Read the model definition and answer for the solid it produces. Units are mm, in the model's axes. Face numbers are marked on the shaded views. A direction names the side the tool comes from. Round coordinates to 2 decimals unless told otherwise and drop trailing zeros. Order: outer loops, then holes, each group sorted by start corner. A loop starts at its lowest first (then second) coordinate and runs counter-clockwise, first axis right, second up. Notation, with made-up numbers: (-20.75, 6.5) - (6.25, 6.5) arc R21 ccw to (6.25, 28.5) - close; hole circle Ø4 at (49.25, 9). An arc over 180 degrees is marked (long way). One line per question, with ' | ' between items. Start each with the question number.
1) The mould has two halves that part along X. Classify the marked faces 6, 7, 8 and 9: pulls with the +X half, pulls with the -X half, needs draft (parallel to the pull), parting line crosses it, or undercut.
2) Flat-ended cylindrical pins translate along their axes: pin 1 (20.5 mm diameter, centred on x = 66.5, y = -26, fed in from -Z); pin 2 (10 mm diameter, centred on x = -58.7, z = 38.1, fed in from -Y) (3 decimals); pin 3 (5 mm diameter, centred on x = -50.5, y = -50, fed in from -Z). Find the tip coordinate at first contact, or state that the pin passes through.
3) The part is cut by section A-A, the plane x = 0. Give the vertices of the cut face in (y, z) (3 decimals), plus the area to 3 significant figures.
4) For the marked faces 1, 2, 3, 4 and 5, determine the directions among +Z, -Z, +X, -X, +Y, -Y from which every point of the face is accessible in a straight line to the end or side of a thin tool.
5) The part is cut by section B-B, the plane z = 0. Give the vertices of the cut face in (x, y) (3 decimals), plus the area to 3 significant figures.
6) The part is cut by section D-D, the plane z = 25. Give the vertices of the cut face in (x, y) (3 decimals).
7) The part is cut by section C-C, the plane y = -20.5. Give the vertices of the cut face in (x, z).
8) Straight lines are drawn through the part: line 1 (X direction, y = -63, z = 38); line 2 (Z direction, x = 67.5, y = -17); line 3 (Y direction, x = -33.5, z = 19.5) (3 decimals). For each, find the intervals that lie inside material, in ascending order. Write a range as from..to.
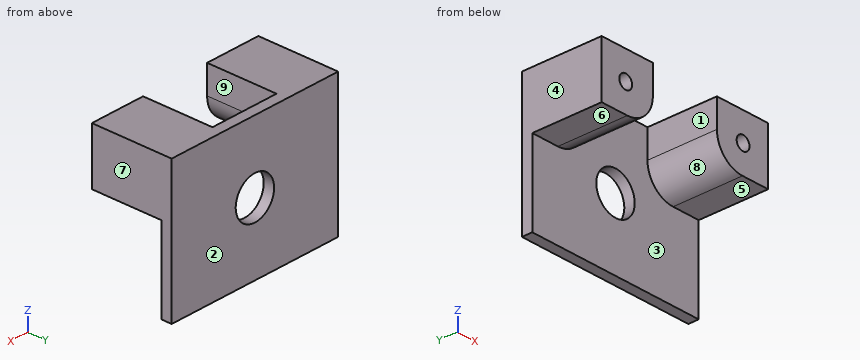
from build123d import *

# Parameters (mm, degrees)
F0_W     = 165.1
F0_H     = 127
F1_DEPTH = 9.525
F3_DEPTH = 63.5
F4_R     = 19.05
F6_DEPTH = 50.8
F5_R     = 6.35
F7_DEPTH = 25.4
F8_R     = 6.35
F9_DEPTH = 25.4


with BuildPart() as f1:
    # F0 (on Front) → F1 (new body)
    with BuildSketch(Plane.XZ):
        Rectangle(F0_W, F0_H)
    extrude(amount=F1_DEPTH)

    # F2 (on face) → F3 (join)
    with BuildSketch(Plane.XZ.offset(9.525)):
        with BuildLine():
            Line((82.55, 63.5), (31.75, 63.5))
            Line((31.75, 63.5), (31.75, 38.1))
            ThreePointArc((31.75, 38.1), (39.189488, 20.139488), (57.15, 12.7))
            Line((57.15, 12.7), (82.55, 12.7))
            Line((82.55, 12.7), (82.55, 63.5))
        make_face()
        with BuildLine():
            Line((-31.75, 63.5), (-82.55, 63.5))
            Line((-82.55, 63.5), (-82.55, 12.7))
            Line((-82.55, 12.7), (-57.15, 12.7))
            ThreePointArc((-57.15, 12.7), (-39.189488, 20.139488), (-31.75, 38.1))
            Line((-31.75, 38.1), (-31.75, 63.5))
        make_face()
    extrude(amount=F3_DEPTH)

    # F4 (on face) → F6 (cut)
    with BuildSketch(Plane.XZ.offset(9.525)):
        Circle(F4_R)
    extrude(amount=-F6_DEPTH, mode=Mode.SUBTRACT)

    # F5 (on face) → F7 (cut)
    with BuildSketch(Plane.XZ.offset(73.025)):
        with Locations((-58.704365, 38.1)):
            Circle(F5_R)
    extrude(amount=-F7_DEPTH, mode=Mode.SUBTRACT)

    # F8 (on face) → F9 (cut)
    with BuildSketch(Plane.XZ.offset(73.025)):
        with Locations((57.692219, 38.1)):
            Circle(F8_R)
    extrude(amount=-F9_DEPTH, mode=Mode.SUBTRACT)


solid = f1.part
Values:
1) face 6: needs draft | face 7: pulls with the +X half | face 8: undercut | face 9: undercut
2) pin 1: stops at z = 12.7 | pin 2: stops at y = -47.625 | pin 3: stops at z = 13.04
3) outline: (-9.525, -63.5) - (0, -63.5) - (0, -19.05) - (-9.525, -19.05) - close; (-9.525, 19.05) - (0, 19.05) - (0, 63.5) - (-9.525, 63.5) - close | area: 847 mm^2
4) face 1: +Z, -Z, -Y | face 2: +Z, -Z, +X, -X, +Y | face 3: -Z, -Y | face 4: +Z, -Z, -X, +Y, -Y | face 5: -Z, +X, -X, -Y
5) outline: (-82.55, -9.525) - (-19.05, -9.525) - (-19.05, 0) - (-82.55, 0) - close; (19.05, -9.525) - (82.55, -9.525) - (82.55, 0) - (19.05, 0) - close | area: 1,210 mm^2
6) outline: (-82.55, -73.025) - (-35.389, -73.025) - (-35.389, -9.525) - (35.389, -9.525) - (35.389, -73.025) - (82.55, -73.025) - (82.55, 0) - (-82.55, 0) - close
7) outline: (-82.55, 12.7) - (-57.15, 12.7) arc R25.4 ccw to (-31.75, 38.1) - (-31.75, 63.5) - (-82.55, 63.5) - close; (31.75, 38.1) arc R25.4 ccw to (57.15, 12.7) - (82.55, 12.7) - (82.55, 63.5) - (31.75, 63.5) - close
8) line 1: x = -82.55..-65.05, -52.36..-31.75, 31.75..51.34, 64.04..82.55 | line 2: z = 12.7..63.5 | line 3: y = -9.525..0
